from build123d import *

# Parameters (mm, degrees)
BOSS_EXTRUDE2_DEPTH = 8.89


with BuildPart() as part:
    # Sketch1 → Boss-Extrude2 (new body)
    with BuildSketch(Plane(origin=(0, 0, 0), x_dir=(1, 0, 0), z_dir=(0, 1, 0))):
        with BuildLine():
            Line((58.42, -19.812), (-58.42, -19.812))
            ThreePointArc((-58.42, -19.812), (-62.012102448, -18.324102448), (-63.5, -14.732))
            Line((-63.5, -14.732), (-63.5, 14.732))
            ThreePointArc((-63.5, 14.732), (-62.012102448, 18.324102448), (-58.42, 19.812))
            Line((-58.42, 19.812), (-14.766931822, 19.812))
            ThreePointArc((-14.766931822, 19.812), (-7.661480975, 20.826090785), (-1.123398019, 23.787388326))
            Line((-1.123398019, 23.787388326), (31.931533802, 44.837295158))
            ThreePointArc((31.931533802, 44.837295158), (40.555754249, 54.042777538), (43.688, 66.261906832))
            Line((43.688, 66.261906832), (43.688, 84.836))
            ThreePointArc((43.688, 84.836), (45.175897552, 88.428102448), (48.768, 89.916))
            Line((48.768, 89.916), (58.42, 89.916))
            ThreePointArc((58.42, 89.916), (62.012102448, 88.428102448), (63.5, 84.836))
            Line((63.5, 84.836), (63.5, 14.732))
            Line((63.5, 14.732), (63.5, -14.732))
            ThreePointArc((63.5, -14.732), (62.012102448, -18.324102448), (58.42, -19.812))
        make_face()
        with BuildLine():
            Line((56.261, 73.787), (56.261, 71.247))
            ThreePointArc((56.261, 71.247), (53.594, 68.58), (50.927, 71.247))
            Line((50.927, 71.247), (50.927, 73.787))
            ThreePointArc((50.927, 73.787), (53.594, 76.454), (56.261, 73.787))
        make_face(mode=Mode.SUBTRACT)
        with BuildLine():
            Line((50.927, 51.054), (50.927, 53.594))
            ThreePointArc((50.927, 53.594), (53.594, 56.261), (56.261, 53.594))
            Line((56.261, 53.594), (56.261, 51.054))
            ThreePointArc((56.261, 51.054), (53.594, 48.387), (50.927, 51.054))
        make_face(mode=Mode.SUBTRACT)
        with BuildLine():
            Line((50.927, 31.369), (50.927, 33.909))
            ThreePointArc((50.927, 33.909), (53.594, 36.576), (56.261, 33.909))
            Line((56.261, 33.909), (56.261, 31.369))
            ThreePointArc((56.261, 31.369), (53.594, 28.702), (50.927, 31.369))
        make_face(mode=Mode.SUBTRACT)
        with BuildLine():
            Line((-54.864, -7.366), (-52.324, -7.366))
            ThreePointArc((-52.324, -7.366), (-49.657, -10.033), (-52.324, -12.7))
            Line((-52.324, -12.7), (-54.864, -12.7))
            ThreePointArc((-54.864, -12.7), (-57.531, -10.033), (-54.864, -7.366))
        make_face(mode=Mode.SUBTRACT)
        with BuildLine():
            Line((54.864, -12.7), (52.324, -12.7))
            ThreePointArc((52.324, -12.7), (49.657, -10.033), (52.324, -7.366))
            Line((52.324, -7.366), (54.864, -7.366))
            ThreePointArc((54.864, -7.366), (57.531, -10.033), (54.864, -12.7))
        make_face(mode=Mode.SUBTRACT)
        with BuildLine():
            Line((-1.27, -7.366), (1.27, -7.366))
            ThreePointArc((1.27, -7.366), (3.937, -10.033), (1.27, -12.7))
            Line((1.27, -12.7), (-1.27, -12.7))
            ThreePointArc((-1.27, -12.7), (-3.937, -10.033), (-1.27, -7.366))
        make_face(mode=Mode.SUBTRACT)
        with BuildLine():
            Line((-54.864, 7.366), (-52.324, 7.366))
            ThreePointArc((-52.324, 7.366), (-49.657, 10.033), (-52.324, 12.7))
            Line((-52.324, 12.7), (-54.864, 12.7))
            ThreePointArc((-54.864, 12.7), (-57.531, 10.033), (-54.864, 7.366))
        make_face(mode=Mode.SUBTRACT)
        with BuildLine():
            Line((54.864, 12.7), (52.324, 12.7))
            ThreePointArc((52.324, 12.7), (49.657, 10.033), (52.324, 7.366))
            Line((52.324, 7.366), (54.864, 7.366))
            ThreePointArc((54.864, 7.366), (57.531, 10.033), (54.864, 12.7))
        make_face(mode=Mode.SUBTRACT)
        with BuildLine():
            Line((-1.27, 7.366), (1.27, 7.366))
            ThreePointArc((1.27, 7.366), (3.937, 10.033), (1.27, 12.7))
            Line((1.27, 12.7), (-1.27, 12.7))
            ThreePointArc((-1.27, 12.7), (-3.937, 10.033), (-1.27, 7.366))
        make_face(mode=Mode.SUBTRACT)
    extrude(amount=BOSS_EXTRUDE2_DEPTH)


solid = part.part
Could you check a few things on this model? Use its own coordinates, in mm. A direction names the side the tool comes from. Coordinates: 2 decimals unless noted, no trailing zeros. Loops run counter-clockwise (first coordinate to the right, second up) from the corner with the lowest first, then second, coordinate; pieces in that order, holes last. Notation, with made-up numbers: (-36.75, -28.75) -> (15.25, -28.75) arc R19 cw to (15.25, -0.75) -> close; hole circle Ø11 at (3, 4.5). An arc over 180 degrees is marked (long way). Answer in a Markdown table with one row per item.
(1) Thinking about a two-plate mould opening in Z: for faces 3 (the face through (61.97, 4.38, -88.47)), 4 (the face through (57.53, 4.38, -9.97)), 5 (the face through (15, 0, -11)), which applies, released by +Z, released by -Z, zero draft, split by the parting line, or undercut?
Results found:
| item | result |
|---|---|
| face 3 | released by -Z |
| face 4 | undercut |
| face 5 | zero draft |
(2) Will these pins go through, and if not, where does the flat tip stop? pin 1 Ø3 at (y, z) = (4, -73) entering from -X; pin 2 Ø3 at (x, y) = (-53.5, 6) entering from -Z; pin 3 Ø3 at (x, y) = (0, 4) entering from -Z.
Results found:
| item | result |
|---|---|
| pin 1 | stops at x = 43.69 |
| pin 2 | stops at z = -19.81 |
| pin 3 | stops at z = -25.46 |
(3) For faces 1 (the face through (3.936, 4.383, 9.974)), 2 (the face through (1, 4, 19.812)), which set-ups out of +Z, -Z, +X, -X, +Y, -Y let a thin tool reach every point of the face, with its end or its side?
Results found:
| item | result |
|---|---|
| face 1 | +Y, -Y |
| face 2 | +Z, +X, -X, +Y, -Y |
(4) Imagine slicing it at C-C (z = -59.5). List the corners of the cut face in (x, y) for me, plus the area to 3 significant figures.
Results found:
| item | result |
|---|---|
| outline | (42.77, 0) -> (63.5, 0) -> (63.5, 8.89) -> (42.77, 8.89) -> close |
| area | 184 mm^2 |
(5) Imagine slicing it at B-B (y = 2.5). Give the number of separate pieces and of enclosed holes in the cut face, plus the area to 3 significant figures.
Results found:
| item | result |
|---|---|
| separate pieces | 1 |
| enclosed holes | 9 |
| area | 6,940 mm^2 |
(6) Imagine slicing it at A-A (x = -37.5). List the corners of the cut face in (y, z) for me, plus the area to 3 significant figures.
Results found:
| item | result |
|---|---|
| outline | (0, -19.81) -> (8.89, -19.81) -> (8.89, 19.81) -> (0, 19.81) -> close |
| area | 352 mm^2 |
(7) If I drill on probe 1 along Z at (x, y) = (-54, 1.5); probe 2 along Z at (x, y) = (-56, 4.75); probe 3 along Z at (x, y) = (-23.5, 2.25), over which ranges is the centre line in solid material (lowest first)?
Results found:
| item | result |
|---|---|
| probe 1 | z = -19.81 to -12.7, -7.37 to 7.37, 12.7 to 19.81 |
| probe 2 | z = -19.81 to -12.45, -7.62 to 7.62, 12.45 to 19.81 |
| probe 3 | z = -19.81 to 19.81 |
